Source: three-view drawing plus pictorial views. Frame: mm from the lowest corner of the part. Give positions to 0.01 mm unless a question says otherwise; leave off trailing zeros. Write each loop counter-clockwise with the first axis right and the second up, starting at its lowest first coordinate (ties: lowest second). Pieces come first, ordered by that corner, then holes. Notation, with made-up numbers: M 55,44 L 68,44 A30 cw 68,69 Z; hole C 59.5,-1 d10. An arc over 180 degrees is marked long. Return JSON: item names as keys, results as strings.
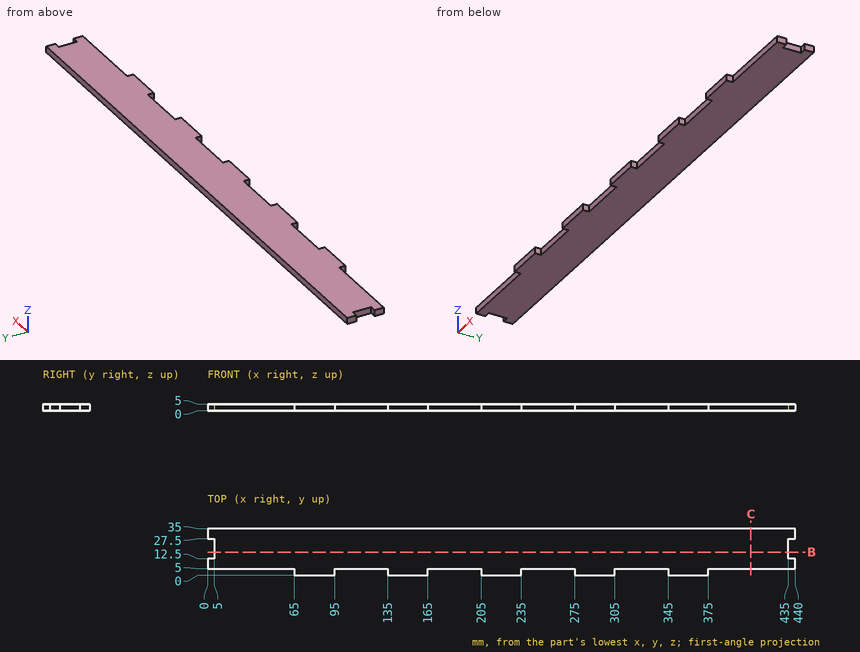
1) Contact query for flat-ended pins moving along their axis: pin 1 Ø2.5 at (y, z) = (3.5, 3.5) entering from +X; pin 2 Ø2.5 at (x, z) = (32.5, 3) entering from -Y; pin 3 Ø1.5 at (y, z) = (3.5, 3.5) entering from -X. Output: stop coordinate, or through.
Numbers:
{"pin 1": "stops at x = 375", "pin 2": "stops at y = 5", "pin 3": "stops at x = 65"}
2) Cut plane C-C, the plane x = 407. Return the cut outline in (y, z).
Numbers:
{"outline": "M 5,0 L 35,0 L 35,5 L 5,5 Z"}
3) Cut plane B-B, the plane y = 17.5. Return the cut outline in (x, z).
Numbers:
{"outline": "M 5,0 L 435,0 L 435,5 L 5,5 Z"}
4) Line query: line 1 (X direction, y = 4.5, z = 3.2); line 2 (Y direction, x = 338.5, z = 0.9); line 3 (X direction, y = 26, z = 2.3). Output: solid intervals per line, ascending. Write a range as [from, to].
Numbers:
{"line 1": "x = [65, 95], [135, 165], [205, 235], [275, 305], [345, 375]", "line 2": "y = [5, 35]", "line 3": "x = [5, 435]"}
